```python
from build123d import *

# Parameters (mm, degrees)
SKETCH1_W                  = 360
SKETCH1_H                  = 250
BASE_FLANGE1_DEPTH         = 3
F_6_0_204_DIAMETER_SLOT1_D = 5.1816
CUT_EXTRUDE1_DEPTH         = 10
CUT_EXTRUDE2_DEPTH         = 10
CUT_EXTRUDE4_DEPTH         = 10
CUT_EXTRUDE5_DEPTH         = 10
CUT_EXTRUDE6_DEPTH         = 10
CUT_EXTRUDE7_DEPTH         = 10
CUT_EXTRUDE8_DEPTH         = 10
EDGE_FLANGE1_DEPTH         = 250


# Sheet-metal steps are written as plain solids
with BuildPart() as part:
    # Sketch1 → Base-Flange1 (new body)
    with BuildSketch(Plane.XY):
        Rectangle(SKETCH1_W, SKETCH1_H)
    extrude(amount=-BASE_FLANGE1_DEPTH)

    # #6 (0.204) Diameter Slot1 (through all)
    with Locations(Plane.XY):
        with Locations((-170, -115), (-170, 115), (170, 115), (170, -115)):
            Hole(F_6_0_204_DIAMETER_SLOT1_D / 2)

    # Sketch8 → Cut-Extrude1 (cut)
    with BuildSketch(Plane.XY):
        with BuildLine():
            Line((-13.5, -113.25), (-6.5, -113.25))
            ThreePointArc((-6.5, -113.25), (-4.75, -115), (-6.5, -116.75))
            Line((-6.5, -116.75), (-13.5, -116.75))
            ThreePointArc((-13.5, -116.75), (-15.25, -115), (-13.5, -113.25))
        make_face()
    extrude(amount=-CUT_EXTRUDE1_DEPTH, mode=Mode.SUBTRACT)

    # Sketch9 → Cut-Extrude2 (cut)
    with BuildSketch(Plane.XY):
        with BuildLine():
            Line((-13.5, 116.75), (-6.5, 116.75))
            ThreePointArc((-6.5, 116.75), (-4.75, 115), (-6.5, 113.25))
            Line((-6.5, 113.25), (-13.5, 113.25))
            ThreePointArc((-13.5, 113.25), (-15.25, 115), (-13.5, 116.75))
        make_face()
    extrude(amount=-CUT_EXTRUDE2_DEPTH, mode=Mode.SUBTRACT)

    # Sketch10 → Cut-Extrude4 (cut)
    with BuildSketch(Plane.XY):
        with BuildLine():
            Line((151.75, 84.5), (151.75, 70.5))
            ThreePointArc((151.75, 70.5), (150, 68.75), (148.25, 70.5))
            Line((148.25, 70.5), (148.25, 84.5))
            ThreePointArc((148.25, 84.5), (150, 86.25), (151.75, 84.5))
        make_face()
    extrude(amount=-CUT_EXTRUDE4_DEPTH, mode=Mode.SUBTRACT)

    # Sketch11 → Cut-Extrude5 (cut)
    with BuildSketch(Plane.XY):
        with BuildLine():
            Line((108, 96.75), (122, 96.75))
            ThreePointArc((122, 96.75), (123.75, 95), (122, 93.25))
            Line((122, 93.25), (108, 93.25))
            ThreePointArc((108, 93.25), (106.25, 95), (108, 96.75))
        make_face()
    extrude(amount=-CUT_EXTRUDE5_DEPTH, mode=Mode.SUBTRACT)

    # Sketch12 → Cut-Extrude6 (cut)
    with BuildSketch(Plane.XY):
        with BuildLine():
            Line((108, 61.75), (122, 61.75))
            ThreePointArc((122, 61.75), (123.75, 60), (122, 58.25))
            Line((122, 58.25), (108, 58.25))
            ThreePointArc((108, 58.25), (106.25, 60), (108, 61.75))
        make_face()
    extrude(amount=-CUT_EXTRUDE6_DEPTH, mode=Mode.SUBTRACT)

    # Sketch13 → Cut-Extrude7 (cut)
    with BuildSketch(Plane.XY):
        with BuildLine():
            Line((81.75, 84.5), (81.75, 70.5))
            ThreePointArc((81.75, 70.5), (80, 68.75), (78.25, 70.5))
            Line((78.25, 70.5), (78.25, 84.5))
            ThreePointArc((78.25, 84.5), (80, 86.25), (81.75, 84.5))
        make_face()
    extrude(amount=-CUT_EXTRUDE7_DEPTH, mode=Mode.SUBTRACT)

    # Sketch14 → Cut-Extrude8 (cut)
    with BuildSketch(Plane.XY):
        with BuildLine():
            Line((-122.5, 30), (-122.5, -30))
            ThreePointArc((-122.5, -30), (-125, -32.5), (-127.5, -30))
            Line((-127.5, -30), (-127.5, 30))
            ThreePointArc((-127.5, 30), (-125, 32.5), (-122.5, 30))
        make_face()
    extrude(amount=-CUT_EXTRUDE8_DEPTH, mode=Mode.SUBTRACT)

    # Edge-Flange1 section (across the edge) → Edge-Flange1 (add)
    with BuildSketch(Plane(origin=(183, -125, 0), x_dir=(-1, 0, 0), z_dir=(0, 1, 0))):
        with BuildLine():
            Line((-3, 3), (-3, 15))
            Line((-3, 15), (0, 15))
            Line((0, 15), (0, 3))
            ThreePointArc((0, 3), (0.878679656, 0.878679656), (3, 0))
            Line((3, 0), (3, -3))
            ThreePointArc((3, -3), (-1.242640687, -1.242640687), (-3, 3))
        make_face()
    extrude(amount=EDGE_FLANGE1_DEPTH)


solid = part.part
```
Check sheet for the modelled part. Datum: model origin and axes. Units: mm. A direction names the side the tool comes from. Round coordinates to 2 decimals unless told otherwise and drop trailing zeros. Write each loop counter-clockwise with the first axis right and the second up, starting at its lowest first coordinate (ties: lowest second). Pieces come first, ordered by that corner, then holes. Notation, with made-up numbers: (25, 1.25) -> (79, 1.25) arc R24 cw to (79, 14.25) -> close; hole circle Ø9 at (6, -35). An arc over 180 degrees is marked (long way). One line per question, with ' | ' between items. Start each with the question number.
1. Sectioned sample at B-B, the plane y = 37.5. Record the cut outline in (x, z), then the cut area to 3 significant figures.
2. Sectioned sample at A-A, the plane y = -12. Record the cut outline in (x, z).
3. Depth check by flat-ended pin: pin 1 (0.9 mm diameter, centred on y = 76, z = -2, fed in from +X); pin 2 (10 mm diameter, centred on x = 73.5, y = 38, fed in from +Z); pin 3 (3 mm diameter, centred on x = 170, y = -115, fed in from -Z); pin 4 (3.5 mm diameter, centred on y = -7, z = -2, fed in from +X). Enter the tip coordinate at first touch or a pass-through.
4. Set-up check for faces 1 (the face through (2, -125, -1)), 2 (the face through (-3, 2, 0)): record each of +Z, -Z, +X, -X, +Y, -Y from which the full face is reachable in a straight line by a thin tool's end or side.
5. Scan lines: line 1 along Y through (x, z) = (-170, -1.25); line 2 along X through (y, z) = (-107.5, 5.5); line 3 along Z through (x, y) = (56, 46). Record each from-to range of solid material in increasing order. Write a range as from..to.
6. Sectioned sample at C-C, the plane z = 8. Record the cut outline in (x, y), then the cut area to 3 significant figures.
7. Sectioned sample at D-D, the plane x = -90. Record the cut outline in (y, z), then the cut area to 3 significant figures.
Taken from the geometry:
1) outline: (-180, -3) -> (180, -3) arc R6 ccw to (186, 3) -> (186, 15) -> (183, 15) -> (183, 3) arc R3 cw to (180, 0) -> (-180, 0) -> close | area: 1,140 mm^2
2) outline: (-180, -3) -> (-127.5, -3) -> (-127.5, 0) -> (-180, 0) -> close; (-122.5, -3) -> (180, -3) arc R6 ccw to (186, 3) -> (186, 15) -> (183, 15) -> (183, 3) arc R3 cw to (180, 0) -> (-122.5, 0) -> close
3) pin 1: stops at x = 183.91 | pin 2: stops at z = 0 | pin 3: passes through | pin 4: stops at x = 185.04
4) face 1: +Z, -Z, +X, -X, -Y | face 2: +Z, -X, +Y, -Y
5) line 1: y = -125..-117.59, -112.41..112.41, 117.59..125 | line 2: x = 183..186 | line 3: z = -3..0
6) outline: (183, -125) -> (186, -125) -> (186, 125) -> (183, 125) -> close | area: 750 mm^2
7) outline: (-125, -3) -> (125, -3) -> (125, 0) -> (-125, 0) -> close | area: 750 mm^2
